Here's how the part is built. I have some questions about the finished solid (model axes, mm). A direction names the side the tool comes from. Round coordinates to 2 decimals unless told otherwise and drop trailing zeros. Write each loop counter-clockwise with the first axis right and the second up, starting at its lowest first coordinate (ties: lowest second). Pieces come first, ordered by that corner, then holes. Notation, with made-up numbers: (-10, 61.5) -> (37, 61.5) arc R13 ccw to (37, 81.5) -> close; hole circle Ø6 at (24.25, -1.5). An arc over 180 degrees is marked (long way). Answer as CSV lines item,"result".
```python
from build123d import *

# Parameters (mm, degrees)
SKETCH_1_W          = 45
SKETCH_1_H          = 50
SKETCH_1_R          = 2.15
SKETCH_1_W_2        = 25
SKETCH_1_H_2        = 30
SKETCH_1_R_2        = 17.5
SKETCH_1_R_3        = 6.75
SKETCH_1_R_4        = 1.6
EXTRUDE_1_DEPTH     = 5
CUT_EXTRUDE_START   = -2
SKETCH_2_R          = 4
SKETCH_2_R_2        = 1.6
SKETCH_2_R_3        = 6.75
CUT_EXTRUDE_1_DEPTH = 2
FILLET_2_R          = 3
FILLET_3_R          = 2


with BuildPart() as part:
    # ｽｹｯﾁ1 → ﾎﾞｽ - 押し出し1 (new body)
    # profile 1 of 4: a face of its own
    with BuildSketch(Plane.XY):
        with Locations((22.5, 25)):
            Rectangle(SKETCH_1_W, SKETCH_1_H)
        with Locations((39.5, 45)):
            Circle(SKETCH_1_R, mode=Mode.SUBTRACT)
        with Locations((5.5, 45)):
            Circle(SKETCH_1_R, mode=Mode.SUBTRACT)
        with Locations((5.5, 5)):
            Circle(SKETCH_1_R, mode=Mode.SUBTRACT)
        with Locations((39.5, 5)):
            Circle(SKETCH_1_R, mode=Mode.SUBTRACT)
        with Locations((22.5, 25)):
            Rectangle(SKETCH_1_W_2, SKETCH_1_H_2, mode=Mode.SUBTRACT)
    # profile 2 of 4: a face of its own
    with BuildSketch(Plane.XY):
        with Locations((67.75, 25)):
            Circle(SKETCH_1_R_2)
        with Locations((67.75, 25)):
            Circle(SKETCH_1_R_3, mode=Mode.SUBTRACT)
        with Locations((67.75, 34.5)):
            Circle(SKETCH_1_R_4, mode=Mode.SUBTRACT)
        with Locations((75.977241336, 20.25)):
            Circle(SKETCH_1_R_4, mode=Mode.SUBTRACT)
        with Locations((59.522758664, 20.25)):
            Circle(SKETCH_1_R_4, mode=Mode.SUBTRACT)
    # profile 3 of 4: a face of its own
    with BuildSketch(Plane.XY):
        with BuildLine():
            Line((72.725574461, 41.77777276), (45, 50))
            Line((45, 50), (45, 39.569533304))
            Line((45, 39.569533304), (54.723538773, 36.685944887))
            ThreePointArc((54.723538773, 36.685944887), (62.987031157, 41.839362452), (72.725574461, 41.77777276))
        make_face()
    # profile 4 of 4: a face of its own
    with BuildSketch(Plane.XY):
        with BuildLine():
            Line((45, 10.430466696), (45, 0))
            Line((45, 0), (72.725574461, 8.22222724))
            ThreePointArc((72.725574461, 8.22222724), (62.987031157, 8.160637548), (54.723538773, 13.314055113))
            Line((54.723538773, 13.314055113), (45, 10.430466696))
        make_face()
    extrude(amount=EXTRUDE_1_DEPTH)

    # ｽｹｯﾁ2 → ｶｯﾄ - 押し出し1 (cut)
    # profile 1 of 6: a face of its own
    with BuildSketch(Plane.XY.offset(5).offset(CUT_EXTRUDE_START)):
        with Locations((67.75, 34.5)):
            Circle(SKETCH_2_R)
        with Locations((67.75, 34.5)):
            Circle(SKETCH_2_R_2, mode=Mode.SUBTRACT)
    # profile 2 of 6: a face of its own
    with BuildSketch(Plane.XY.offset(5).offset(CUT_EXTRUDE_START)):
        with Locations(Location((67.75, 25, 0), (0, 0, 189.100972034))):
            Circle(SKETCH_2_R_3)
    # profile 3 of 6: a face of its own
    with BuildSketch(Plane.XY.offset(5).offset(CUT_EXTRUDE_START)):
        with Locations(Location((67.75, 25, 0), (0, 0, 189.100972034))):
            Circle(SKETCH_2_R_3)
    # profile 4 of 6: a face of its own
    with BuildSketch(Plane.XY.offset(5).offset(CUT_EXTRUDE_START)):
        with Locations((59.522758664, 20.25)):
            Circle(SKETCH_2_R)
        with Locations((59.522758664, 20.25)):
            Circle(SKETCH_2_R_2, mode=Mode.SUBTRACT)
    # profile 5 of 6: a face of its own
    with BuildSketch(Plane.XY.offset(5).offset(CUT_EXTRUDE_START)):
        with Locations(Location((67.75, 25, 0), (0, 0, 189.100972034))):
            Circle(SKETCH_2_R_3)
    # profile 6 of 6: a face of its own
    with BuildSketch(Plane.XY.offset(5).offset(CUT_EXTRUDE_START)):
        with Locations((75.977241336, 20.25)):
            Circle(SKETCH_2_R)
        with Locations((75.977241336, 20.25)):
            Circle(SKETCH_2_R_2, mode=Mode.SUBTRACT)
    extrude(amount=CUT_EXTRUDE_1_DEPTH, mode=Mode.SUBTRACT)

    # ﾌｨﾚｯﾄ2
    fillet_2_edges = [part.edges().sort_by_distance(p)[0] for p in [
        (35, 40, 2.5),
        (10, 40, 2.5),
        (10, 10, 2.5),
        (35, 10, 2.5),
        (45, 39.569533304, 2.5),
        (45, 10.430466696, 2.5),
        (54.723538773, 13.314055113, 2.5),
        (54.723538773, 36.685944887, 2.5),
    ]]
    fillet(fillet_2_edges, radius=FILLET_2_R)

    # ﾌｨﾚｯﾄ3
    fillet_3_edges = [part.edges().sort_by_distance(p)[0] for p in [
        (0, 0, 2.5),
        (0, 50, 2.5),
    ]]
    fillet(fillet_3_edges, radius=FILLET_3_R)


solid = part.part
```
1. Suppose I cut it at C-C on y = 45. Please give me the cut outline in (x, z).
Numbers:
outline,"(0, 0) -> (3.35, 0) -> (3.35, 5) -> (0, 5) -> close; (7.65, 0) -> (37.35, 0) -> (37.35, 5) -> (7.65, 5) -> close; (41.65, 0) -> (61.86, 0) -> (61.86, 5) -> (41.65, 5) -> close"
2. If I drill on line 1 (Y direction, x = 39.5, z = 1.9); line 2 (Y direction, x = 28, z = 2.45); line 3 (X direction, y = 23, z = 4.3), over which ranges is the centre line in solid material (lowest first)?
Numbers:
line 1,"y = 0 to 2.85, 7.15 to 42.85, 47.15 to 50"
line 2,"y = 0 to 10, 40 to 50"
line 3,"x = 0 to 10, 35 to 45, 50.36 to 56.62, 78.88 to 85.14"
3. Suppose I cut it at B-B on z = 0.95. Count the separate pieces of the cut face and the enclosed holes in it, and give its area (3 significant figures).
Numbers:
separate pieces,"1"
enclosed holes,"10"
area,"2,580 mm^2"
4. If we mould it in two halves opening along Y, with no side actions, what happens to faces 4 (the face through (52.648, 13.904, 2.535)), 5 (the face through (59.06, 45.83, 2.46)), 6 (the face through (85.247, 24.686, 2.465)), 7 (the face through (45, 25, 2))? For each: released by +Y, released by -Y, zero draft, split by the parting line, or undercut.
Numbers:
face 4,"undercut"
face 5,"released by +Y"
face 6,"split by the parting line"
face 7,"undercut"
5. For pin 1 Ø2.5 at (y, z) = (27, 1.5) entering from +X, with a flat end and sliding along its axis, tell me the tip position at first contact or that it passes through.
Numbers:
pin 1,"stops at x = 85.23"
6. Suppose I cut it at D-D on x = 21. Please give me the cut outline in (y, z), and give its area (3 significant figures).
Numbers:
outline,"(0, 0) -> (10, 0) -> (10, 5) -> (0, 5) -> close; (40, 0) -> (50, 0) -> (50, 5) -> (40, 5) -> close"
area,"100 mm^2"
7. On a 3-axis mill with a long thin cutter (end or side, diameter ignored), from which of +Z, -Z, +X, -X, +Y, -Y can I reach the whole of each face in a straight line? I mean faces 1 (the face through (10.9, 39.14, 2.54)), 2 (the face through (66, 35, 3)), 3 (the face through (42, 25, 5)). Say none if no direction works.
Numbers:
face 1,"+Z, -Z"
face 2,"+Z"
face 3,"+Z, +X, -X, +Y, -Y"
8. Suppose I cut it at A-A on x = 5.5. Please give me the cut outline in (y, z).
Numbers:
outline,"(0, 0) -> (2.85, 0) -> (2.85, 5) -> (0, 5) -> close; (7.15, 0) -> (42.85, 0) -> (42.85, 5) -> (7.15, 5) -> close; (47.15, 0) -> (50, 0) -> (50, 5) -> (47.15, 5) -> close"
